Design review of the part built by this model. Coordinates are the model's own, in mm. A direction names the side the tool comes from. Coordinates: 2 decimals unless noted, no trailing zeros. Loops run counter-clockwise (first coordinate to the right, second up) from the corner with the lowest first, then second, coordinate; pieces in that order, holes last.
Q1. For P1, Ø3, axis at x = 9, z = -1, coming from the +Y side; P2, Ø10, axis at x = -4.5, y = -12.5, coming from the +Z side; P3, Ø2, axis at x = -9, z = -1, coming from the -Y side; P4, Ø6, axis at x = -1, z = -3.5, coming from the -Y side, all flat-tipped, find the tip position at first contact; note any pin that passes through.
Q2. Draft analysis for pull direction Z (two halves, no side actions). For faces 6 (the face through (0, -11, 12)), 7 (the face through (0, -22, 10)), 8 (the face through (9.845, 1.014, -12.921)), state which applies: released by +Z, released by -Z, zero draft, split by the parting line, or undercut.
Q3. Add section C-C on x = 0. Give the boundary of the cut face in (y, z), and give its area (3 significant figures).
Q4. Add section D-D on z = -6.5. Give the boundary of the cut face in (x, y), and give its area (3 significant figures).
Q5. Machinability: for faces 1 (the face through (0, 1, 14)), 2 (the face through (0, -11, 7)), 3 (the face through (-10.25, -11, 9)), 4 (the face through (-10.24, 1.01, -11.84)), 5 (the face through (10.25, -11, 9)), which of the approach directions +Z, -Z, +X, -X, +Y, -Y give a long, thin tool a straight path to every point of the face, cutting with its end or side? Answer none if there is none.
Q6. Add section B-B on z = -1. Give the boundary of the cut face in (x, y), and give its area (3 significant figures).
Q7. Wall thickness on probe 1 along X at (y, z) = (1.45, -12); probe 2 along Z at (x, y) = (-9, 1.25); probe 3 along X at (y, z) = (1.15, -6.5): over which ranges is each line inside the solid? List them lowest first.
Q8. Add section A-A on x = -9. Give the boundary of the cut face in (y, z), and give its area (3 significant figures).
```python
from build123d import *

# Parameters (mm, degrees)
SKETCH_1_W                      = 22
SKETCH_1_H                      = 28
EXTRUDE_1_DEPTH                 = 2
CUT_EXTRUDE_1_REACH             = 19.916
SKETCH_2_R                      = 1.25
SKETCH_3_W                      = 20.5
SKETCH_3_H                      = 5
EXTRUDE_2_DEPTH                 = 22
CUT_EXTRUDE_2_REACH             = 31.883
SKETCH_4_R                      = 1
CUT_EXTRUDE_2_DIRECTION_2_DEPTH = 30.883105595


with BuildPart() as part:
    # 草图1 → 凸台-拉伸1 (new body)
    with BuildSketch(Plane(origin=(0, 0, 0), x_dir=(1, 0, 0), z_dir=(0, 1, 0))):
        Rectangle(SKETCH_1_W, SKETCH_1_H)
    extrude(amount=EXTRUDE_1_DEPTH)

    # 草图2 → 切除-拉伸1 (cut, up to next)
    with BuildSketch(Plane(origin=(0, 2, 0), x_dir=(1, 0, 0), z_dir=(0, 1, 0)), mode=Mode.PRIVATE) as cut_extrude_1_sk1:
        with Locations(Location((9, 12, 0), (0, 0, 270))):
            Circle(SKETCH_2_R)
    cut_extrude_1_tool1 = extrude(cut_extrude_1_sk1.sketch, amount=-CUT_EXTRUDE_1_REACH, mode=Mode.PRIVATE) & part.part
    # 草图2 → 切除-拉伸1 (cut, up to next)
    with BuildSketch(Plane(origin=(0, 2, 0), x_dir=(1, 0, 0), z_dir=(0, 1, 0)), mode=Mode.PRIVATE) as cut_extrude_1_sk2:
        with Locations(Location((-9, 12, 0), (0, 0, 90))):
            Circle(SKETCH_2_R)
    cut_extrude_1_tool2 = extrude(cut_extrude_1_sk2.sketch, amount=-CUT_EXTRUDE_1_REACH, mode=Mode.PRIVATE) & part.part
    # 草图2 → 切除-拉伸1 (cut, up to next)
    with BuildSketch(Plane(origin=(0, 2, 0), x_dir=(1, 0, 0), z_dir=(0, 1, 0)), mode=Mode.PRIVATE) as cut_extrude_1_sk3:
        with Locations(Location((-9, 1, 0), (0, 0, 90))):
            Circle(SKETCH_2_R)
    cut_extrude_1_tool3 = extrude(cut_extrude_1_sk3.sketch, amount=-CUT_EXTRUDE_1_REACH, mode=Mode.PRIVATE) & part.part
    # 草图2 → 切除-拉伸1 (cut, up to next)
    with BuildSketch(Plane(origin=(0, 2, 0), x_dir=(1, 0, 0), z_dir=(0, 1, 0)), mode=Mode.PRIVATE) as cut_extrude_1_sk4:
        with Locations(Location((9, 1, 0), (0, 0, 270))):
            Circle(SKETCH_2_R)
    cut_extrude_1_tool4 = extrude(cut_extrude_1_sk4.sketch, amount=-CUT_EXTRUDE_1_REACH, mode=Mode.PRIVATE) & part.part
    add(cut_extrude_1_tool1.solids().sort_by_distance((9, 2, -12))[0], mode=Mode.SUBTRACT)
    add(cut_extrude_1_tool2.solids().sort_by_distance((-9, 2, -12))[0], mode=Mode.SUBTRACT)
    add(cut_extrude_1_tool3.solids().sort_by_distance((-9, 2, -1))[0], mode=Mode.SUBTRACT)
    add(cut_extrude_1_tool4.solids().sort_by_distance((9, 2, -1))[0], mode=Mode.SUBTRACT)

    # 草图3 → 凸台-拉伸2 (add)
    with BuildSketch(Plane.XZ):
        with Locations((0, 9.5)):
            Rectangle(SKETCH_3_W, SKETCH_3_H)
    extrude(amount=EXTRUDE_2_DEPTH)

    # 草图4 → 切除-拉伸2 (cut, up to next)
    with BuildSketch(Plane(origin=(0, 2, 0), x_dir=(1, 0, 0), z_dir=(0, 1, 0)), mode=Mode.PRIVATE) as cut_extrude_2_sk1:
        with Locations(Location((0, 6.5, 0), (0, 0, 90))):
            Circle(SKETCH_4_R)
    cut_extrude_2_tool1 = extrude(cut_extrude_2_sk1.sketch, amount=-CUT_EXTRUDE_2_REACH, mode=Mode.PRIVATE) & part.part
    add(cut_extrude_2_tool1.solids().sort_by_distance((0, 2, -6.5))[0], mode=Mode.SUBTRACT)

    # 草图4 → 切除-拉伸2 direction 2 (cut)
    with BuildSketch(Plane(origin=(0, 2, 0), x_dir=(1, 0, 0), z_dir=(0, 1, 0))):
        with Locations(Location((0, 6.5, 0), (0, 0, 90))):
            Circle(SKETCH_4_R)
    extrude(amount=CUT_EXTRUDE_2_DIRECTION_2_DEPTH, mode=Mode.SUBTRACT)


solid = part.part
```
Entries:
1. P1: stops at y = 2
1. P2: stops at z = 12
1. P3: passes through
1. P4: stops at y = 0
2. face 6: released by +Z
2. face 7: zero draft
2. face 8: undercut
3. outline: (-22, 7) - (0, 7) - (0, -5.5) - (2, -5.5) - (2, 14) - (0, 14) - (0, 12) - (-22, 12) - close; (0, -14) - (2, -14) - (2, -7.5) - (0, -7.5) - close
3. area: 162 mm2
4. outline: (-11, 0) - (-1, 0) - (-1, 2) - (-11, 2) - close; (1, 0) - (11, 0) - (11, 2) - (1, 2) - close
4. area: 40.0 mm2
5. face 1: +Z, +X, -X, +Y, -Y
5. face 2: -Z, +X, -X, -Y
5. face 3: +Z, -Z, -X, -Y
5. face 4: +Y, -Y
5. face 5: +Z, -Z, +X, -Y
6. outline: (-11, 0) - (-10.25, 0) - (-10.25, 2) - (-11, 2) - close; (-7.75, 0) - (7.75, 0) - (7.75, 2) - (-7.75, 2) - close; (10.25, 0) - (11, 0) - (11, 2) - (10.25, 2) - close
6. area: 34.0 mm2
7. probe 1: x = -11 to -10.25, -7.75 to 7.75, 10.25 to 11
7. probe 2: z = -14 to -13.25, -10.75 to -2.25, 0.25 to 14
7. probe 3: x = -11 to -1, 1 to 11
8. outline: (-22, 7) - (0, 7) - (0, 0.25) - (2, 0.25) - (2, 14) - (0, 14) - (0, 12) - (-22, 12) - close; (0, -14) - (2, -14) - (2, -13.25) - (0, -13.25) - close; (0, -10.75) - (2, -10.75) - (2, -2.25) - (0, -2.25) - close
8. area: 156 mm2
